Geometry check sheet. Reference: the model listing, model coordinates, mm. Face numbers are marked on the shaded views. A direction names the side the tool comes from. Give positions to 0.01 mm unless a question says otherwise; leave off trailing zeros. Write each loop counter-clockwise with the first axis right and the second up, starting at its lowest first coordinate (ties: lowest second). Pieces come first, ordered by that corner, then holes. Notation, with made-up numbers: (-17.75, -34.5) - (16.25, -34.5) arc R16 cw to (16.25, -29.5) - close; hole circle Ø4 at (1.5, -21). An arc over 180 degrees is marked (long way). Write item = value, one per line. Start each with the question number.
(1) Section check B-B, the plane z = 11. Enter the section's corners in (x, y), plus the area to 3 significant figures.
(2) Draft check along Z on the marked faces 1, 2, 3 and 4. Enter one of: pulls with the +Z half, pulls with the -Z half, needs draft (parallel to the pull), parting line crosses it, or undercut.
(3) Section check C-C, the plane y = 28. Enter the section's corners in (x, z), plus the area to 3 significant figures.
(4) Access from +Z, -Z, +X, -X, +Y, -Y to the whole of each face (thin tool, end or side, straight path). Record for the marked faces 5, 6 and 7.
(5) Section check D-D, the plane z = 23. Enter the section's corners in (x, y), plus the area to 3 significant figures.
(6) Thickness scan on L1, parallel to Z at x = 13.5, y = 26; L2, parallel to X at y = 26.75, z = 36.4; L3, parallel to Y at x = 10, z = 3.5. Record the ranges inside material, lowest first.
(7) Section check A-A, the plane x = 13.5. Enter the section's corners in (y, z), plus the area to 3 significant figures.
(8) Depth check by flat-ended pin: pin 1 Ø5 at (y, z) = (20.5, 17) entering from +X; pin 2 Ø4 at (x, z) = (18.5, 20.5) entering from +Y; pin 3 Ø5 at (x, y) = (12, 7.5) entering from +Z; pin 4 Ø0.9 at (y, z) = (29.5, 7) entering from -X. Enter the tip coordinate at first touch or a pass-through.
Autodesk Inventor part; units mm, degrees
ref_plane "YZ Plane" through (0, 0, 0) normal (1, 0, 0) x (0, 1, 0)
ref_plane "XZ Plane" through (0, 0, 0) normal (0, 1, 0) x (-1, 0, 0)
ref_plane "XY Plane" through (0, 0, 0) normal (0, 0, 1) x (1, 0, 0)
sketch "Sketch1" plane through (0, 0, 0) normal (0, 0, 1) x (1, 0, 0)
  line L0 (0, 0) -> (27, 0)
  line L1 (27, 0) -> (27, 29)
  line L2 (27, 29) -> (0, 29)
  line L3 (0, 29) -> (0, 0)
  dimension "d0" = 27
  dimension "d1" = 29
extrude "Extrusion1" add sketch "Sketch1" along normal blind 4
sketch "Sketch2" plane through (0, 0, 4) normal (0, 0, 1) x (1, 0, 0)
  line L0 (27, 29) -> (0, 29)
  point P0 (0, 0)
  point P1 (2.5, 20.5)
  point P2 (24.5, 20.5)
  point P3 (2.5, 8.5)
  point P4 (24.5, 8.5)
  dimension "d30" = 8.5
  dimension "d31" = 12
  dimension "d32" = 8.5
  dimension "d33" = 12
sketch "Sketch3" plane through (0, 0, 0) normal (0, 0, -1) x (-1, 0, 0)
  line L0 (0, 29) -> (0, 0)
  point P0 (-13.5, 33)
  point P1 (-13.5, 5)
  dimension "d19" = 13.5
  dimension "d20" = 13.5
sketch "Sketch6" plane through (0, 0, 4) normal (0, 0, 1) x (1, 0, 0)
  line L0 (0, 29) -> (0, 0)
  line L1 (27, 0) -> (27, 29)
  line L2 (0, 29) -> (27, 29)
  line L3 (27, 29) -> (27, 24)
  line L4 (27, 24) -> (0, 24)
  line L5 (0, 24) -> (0, 29)
  dimension "d34" = 5
extrude "Extrusion4" add sketch "Sketch6" along normal blind 38.4
sketch "Sketch8" plane through (0, 29, 0) normal (0, 1, 0) x (1, 0, 0)
  line L0 (0, 0) -> (27, 0)
  line L1 (0, -42.4) -> (27, -42.4)
  line L2 (10.35, 0) -> (16.65, 0)
  line L3 (16.65, 0) -> (16.65, -42.4)
  line L4 (16.65, -42.4) -> (10.35, -42.4)
  line L5 (10.35, -42.4) -> (10.35, 0)
  line L6 (0, 0) -> (0, -42.4)
  dimension "d41" = 6.3
  dimension "d51" = 10.35
extrude "Extrusion6" add sketch "Sketch8" along normal blind 1.5 contours L0 L3 L1 L5
sketch "Sketch9" plane through (0, 24, 4) normal (0, -1, 0) x (1, 0, 0)
  line L0 (0, 0) -> (27, 0)
  point P0 (0, -4)
  point P1 (13.5, 7)
  point P2 (13.5, 20)
  dimension "d69" = 7
hole "Hole3" at (13.5, 24, 11) direction (0, 1, 0) diameter 6.6 end through all
fillet "Fillet1" radius 2 1 edges at (13.5, 24, 4)
sketch "Sketch10" plane through (0, 0, 4) normal (0, 0, 1) x (1, 0, 0)
  line L0 (24.5, 20.9) -> (24.5, 20.1) construction
  line L1 (23.4, 20.9) -> (23.4, 20.1)
  line L2 (25.6, 20.1) -> (25.6, 20.9)
  arc A0 (25.6, 20.9) -> (23.4, 20.9) centre (24.5, 20.9) ccw
  arc A1 (23.4, 20.1) -> (25.6, 20.1) centre (24.5, 20.1) ccw
  line L3 (24.5, 8.9) -> (24.5, 8.1) construction
  line L4 (23.4, 8.9) -> (23.4, 8.1)
  line L5 (25.6, 8.1) -> (25.6, 8.9)
  arc A2 (25.6, 8.9) -> (23.4, 8.9) centre (24.5, 8.9) ccw
  arc A3 (23.4, 8.1) -> (25.6, 8.1) centre (24.5, 8.1) ccw
  line L6 (2.5, 20.9) -> (2.5, 20.1) construction
  line L7 (1.4, 20.9) -> (1.4, 20.1)
  line L8 (3.6, 20.1) -> (3.6, 20.9)
  arc A4 (3.6, 20.9) -> (1.4, 20.9) centre (2.5, 20.9) ccw
  arc A5 (1.4, 20.1) -> (3.6, 20.1) centre (2.5, 20.1) ccw
  line L9 (2.5, 8.1) -> (2.5, 8.9) construction
  line L10 (3.6, 8.1) -> (3.6, 8.9)
  line L11 (1.4, 8.9) -> (1.4, 8.1)
  arc A6 (1.4, 8.1) -> (3.6, 8.1) centre (2.5, 8.1) ccw
  arc A7 (3.6, 8.9) -> (1.4, 8.9) centre (2.5, 8.9) ccw
  point P0 (0, 0)
  point P1 (24.5, 20.5)
  point P2 (24.5, 8.5)
  point P3 (2.5, 20.5)
  point P4 (2.5, 8.5)
  dimension "d53" = 0.4
  dimension "d54" = 2.2
  dimension "d55" = 0.4
  dimension "d56" = 2.2
  dimension "d57" = 0.4
  dimension "d58" = 2.2
  dimension "d59" = 0.4
  dimension "d60" = 2.2
extrude "Extrusion7" cut sketch "Sketch10" against normal through all
chamfer "Chamfer1" distance 0.4 angle 45 1 edges at (16.65, 30.5, 27.1918)
chamfer "Chamfer2" distance 0.4 angle 45 3 edges at (16.65, 30.5, 5.0082) (10.35, 30.5, 27.1918) (10.35, 30.5, 5.0082)
sketch "Sketch11" plane through (0, 24, 42.4) normal (0, -1, 0) x (1, 0, 0)
  point P0 (0, -42.4)
  point P1 (13.5, -6)
hole "Hole4" at (13.5, 24, 36.4) direction (0, 1, 0) diameter 6.6 end through all
properties part number "CameraMountA"
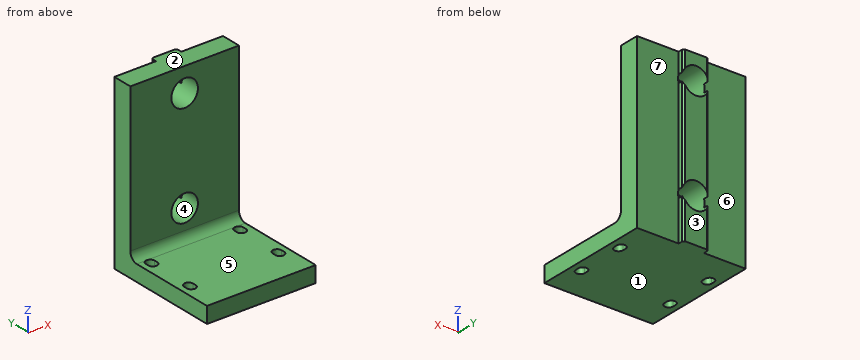
Model answer:
q1.outline = (0, 24) - (10.2, 24) - (10.2, 29) - (0, 29) - close; (16.8, 24) - (27, 24) - (27, 29) - (16.8, 29) - close
q1.area = 102 mm²
q2.face_1 = pulls with the -Z half
q2.face_2 = pulls with the +Z half
q2.face_3 = needs draft
q2.face_4 = undercut
q3.outline = (0, 0) - (27, 0) - (27, 42.4) - (0, 42.4) - close; hole circle Ø6.6 at (13.5, 11); hole circle Ø6.6 at (13.5, 36.4)
q3.area = 1,080 mm²
q4.face_5 = +Z, +X, -X, -Y
q4.face_6 = +Z, -Z, -X, +Y
q4.face_7 = +Z, -Z, +X, +Y
q5.outline = (0, 24) - (27, 24) - (27, 29) - (16.65, 29) - (16.65, 30.1) - (16.25, 30.5) - (10.75, 30.5) - (10.35, 30.1) - (10.35, 29) - (0, 29) - close
q5.area = 144 mm²
q6.L1 = 0 to 7.7, 14.3 to 33.1, 39.7 to 42.4
q6.L2 = 0 to 10.2, 16.8 to 27
q6.L3 = 0 to 29
q7.outline = (0, 0) - (30.5, 0) - (30.5, 7.7) - (24, 7.7) - (24, 6) arc R2 cw to (22, 4) - (0, 4) - close; (24, 14.3) - (30.5, 14.3) - (30.5, 33.1) - (24, 33.1) - close; (24, 39.7) - (30.5, 39.7) - (30.5, 42.4) - (24, 42.4) - close
q7.area = 287 mm²
q8.pin_1 = through
q8.pin_2 = 30.25
q8.pin_3 = 4
q8.pin_4 = 10.35
